Could you check a few things on this drawing? It's one solid part, dimensions in mm from its lowest x, y, z. A direction names the side the tool comes from. Coordinates: 2 decimals unless noted, no trailing zeros. Write each loop counter-clockwise with the first axis right and the second up, starting at its lowest first coordinate (ties: lowest second). Pieces come first, ordered by that corner, then holes. Notation, with made-up numbers: M 10,53 L 41,53 A19 ccw 41,65 Z; hole C 81,54.5 d6. An arc over 180 degrees is marked long. Use a Markdown table: item, result.
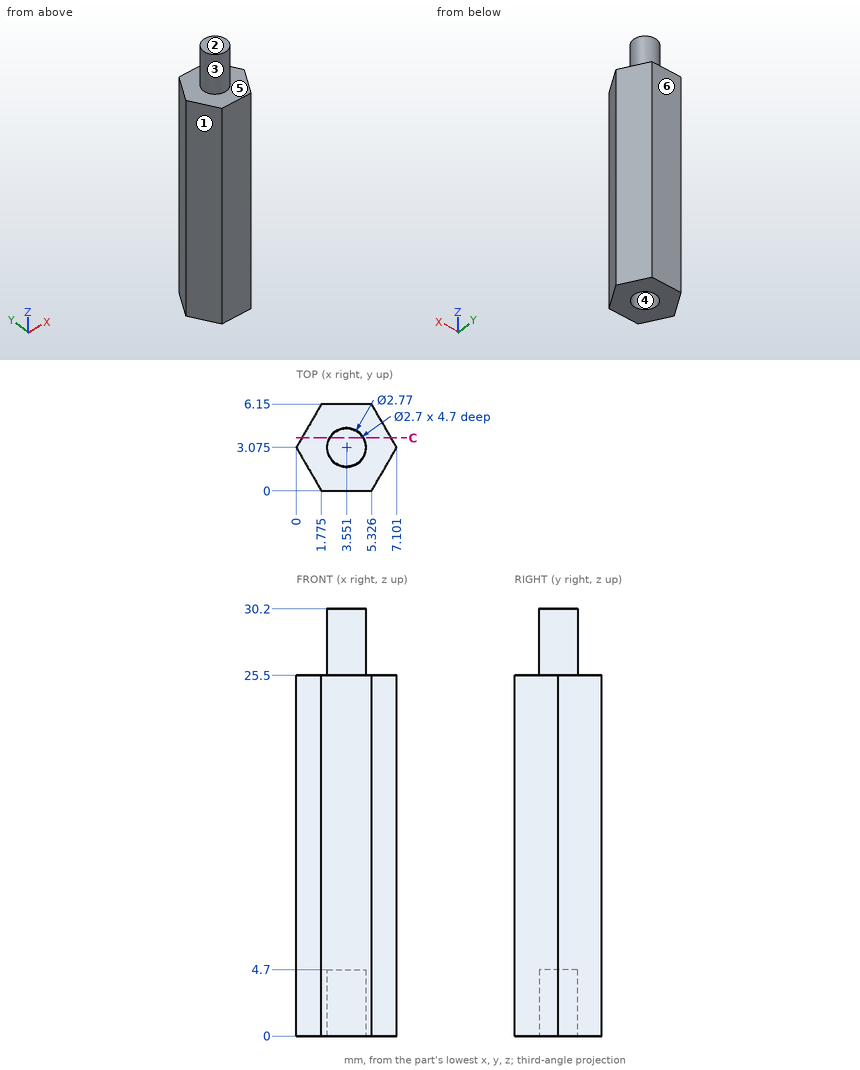
1. We'd pull the mould along Y, two halves only. Please class the marked faces 1, 2, 3 and 4: +Y half, -Y half, draft (parallel to the pull), parting line (faces both ways), or undercut.
Answers follow:
| item | result |
|---|---|
| face 1 | -Y half |
| face 2 | draft |
| face 3 | parting line |
| face 4 | undercut |
2. Suppose I cut it at C-C on y = 3.75. Write out the boundary of the cut face in (x, z), and give its area (3 significant figures).
Answers follow:
| item | result |
|---|---|
| outline | M 0.39,0 L 2.38,0 L 2.38,4.7 L 4.72,4.7 L 4.72,0 L 6.71,0 L 6.71,25.5 L 4.76,25.5 L 4.76,30.2 L 2.34,30.2 L 2.34,25.5 L 0.39,25.5 Z |
| area | 162 mm2 |
3. I need wall thicknesses on probe 1 along Y at (x, z) = (3.5, 26); probe 2 along Z at (x, y) = (3.75, 0.5); probe 3 along Y at (x, z) = (3.25, 27.5). Which ranges of each line are inside material? Lowest first, please.
Answers follow:
| item | result |
|---|---|
| probe 1 | y = 1.69 to 4.46 |
| probe 2 | z = 0 to 25.5 |
| probe 3 | y = 1.72 to 4.43 |
4. Will these pins go through, and if not, where does the flat tip stop? pin 1 Ø1.6 at (x, y) = (3.55, 3.08) entering from -Z; pin 2 Ø1 at (y, z) = (4.5, 20) entering from +X; pin 3 Ø1 at (y, z) = (5.5, 19) entering from -X.
Answers follow:
| item | result |
|---|---|
| pin 1 | stops at z = 4.7 |
| pin 2 | stops at x = 6.57 |
| pin 3 | stops at x = 1.11 |
5. Which directions (+Z, -Z, +X, -X, +Y, -Y) give clear straight access to the entire face, cutting with the end or side of a thin tool? Please do the marked faces 5 and 6.
Answers follow:
| item | result |
|---|---|
| face 5 | +Z |
| face 6 | +Z, -Z, +X, -X, +Y |
